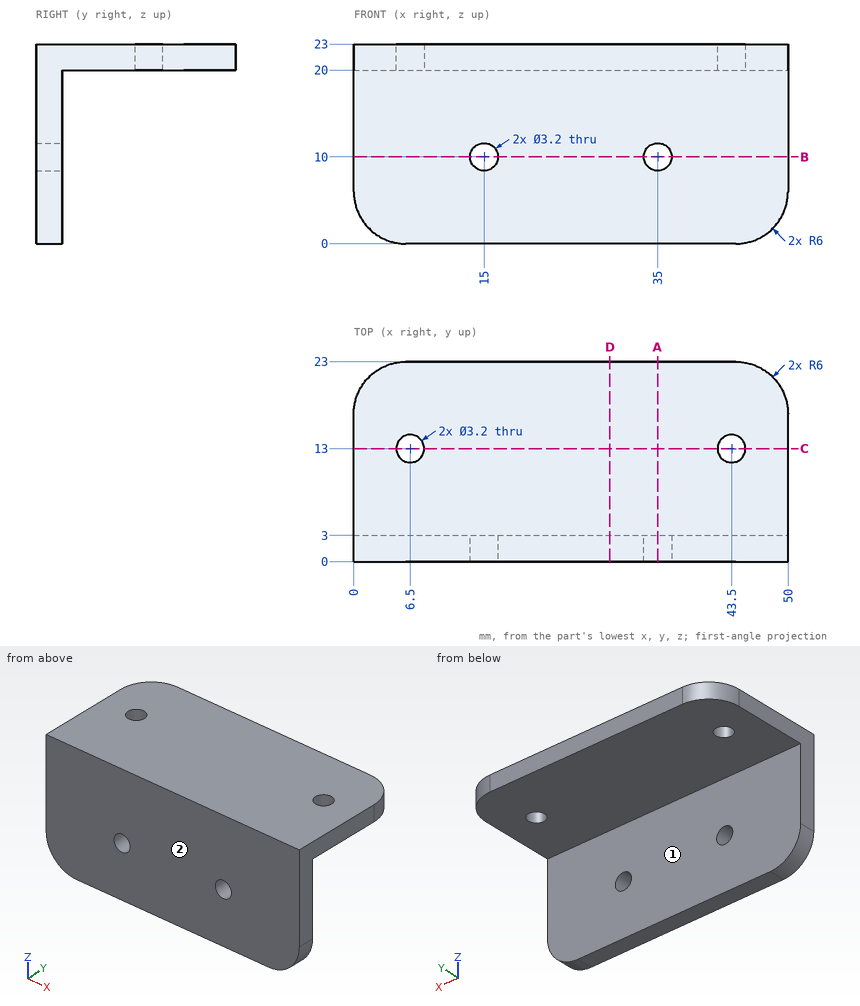
Geometry: see drawing. Coordinates: mm, zero at the bounding-box minimum. A direction names the side the tool comes from. Round coordinates to 2 decimals unless told otherwise and drop trailing zeros. Write each loop counter-clockwise with the first axis right and the second up, starting at its lowest first coordinate (ties: lowest second). Pieces come first, ordered by that corner, then holes. Notation, with made-up numbers: M -29,61 L -22,61 A27 ccw -22,90 Z; hole C 40.25,25.25 d10. An arc over 180 degrees is marked long. Answer as a JSON object with one key per item and string values. Group by question number.
(1) Section query D-D on x = 29.5. Output: boundary loops of the cut face in (y, z).
(2) Section query A-A on x = 35. Output: boundary loops of the cut face in (y, z).
(3) Reachability of the marked faces 1 and 2 from +Z, -Z, +X, -X, +Y, -Y: full face, straight path, thin tool, end or side. Return the list, or none.
(4) First-contact query: pin 1 (1 mm diameter, centred on x = 38, z = 14.5, fed in from +Y); pin 2 (3 mm diameter, centred on y = 3, z = 4, fed in from +X). Flat tips, straight axial feed; report the tip coordinate or a pass-through.
(5) Ray query, line 1 (X direction, y = 1.05, z = 10); line 2 (Y direction, x = 43.5, z = 20.7); line 3 (Z direction, x = 35, y = 1.45). Return the intervals inside material, ascending. Write a range as [from, to].
(6) Section query C-C on y = 13. Output: boundary loops of the cut face in (x, z), then the cut area to 3 significant figures.
(7) Section query B-B on z = 10. Output: boundary loops of the cut face in (x, y).
Computed values:
{
 "1": {"outline": "M 0,0 L 3,0 L 3,20 L 23,20 L 23,23 L 0,23 Z"},
 "2": {"outline": "M 0,0 L 3,0 L 3,8.4 L 0,8.4 Z; M 0,11.6 L 3,11.6 L 3,20 L 23,20 L 23,23 L 0,23 Z"},
 "3": {"face 1": "-Z, +X, -X, +Y", "face 2": "+Z, -Z, +X, -X, -Y"},
 "4": {"pin 1": "y = 3", "pin 2": "x = 49.98"},
 "5": {"line 1": "[0, 13.4], [16.6, 33.4], [36.6, 50]", "line 2": "[0, 11.4], [14.6, 23]", "line 3": "[0, 8.4], [11.6, 23]"},
 "6": {"outline": "M 0,20 L 4.9,20 L 4.9,23 L 0,23 Z; M 8.1,20 L 41.9,20 L 41.9,23 L 8.1,23 Z; M 45.1,20 L 50,20 L 50,23 L 45.1,23 Z", "area": "131 mm^2"},
 "7": {"outline": "M 0,0 L 13.4,0 L 13.4,3 L 0,3 Z; M 16.6,0 L 33.4,0 L 33.4,3 L 16.6,3 Z; M 36.6,0 L 50,0 L 50,3 L 36.6,3 Z"}
}
